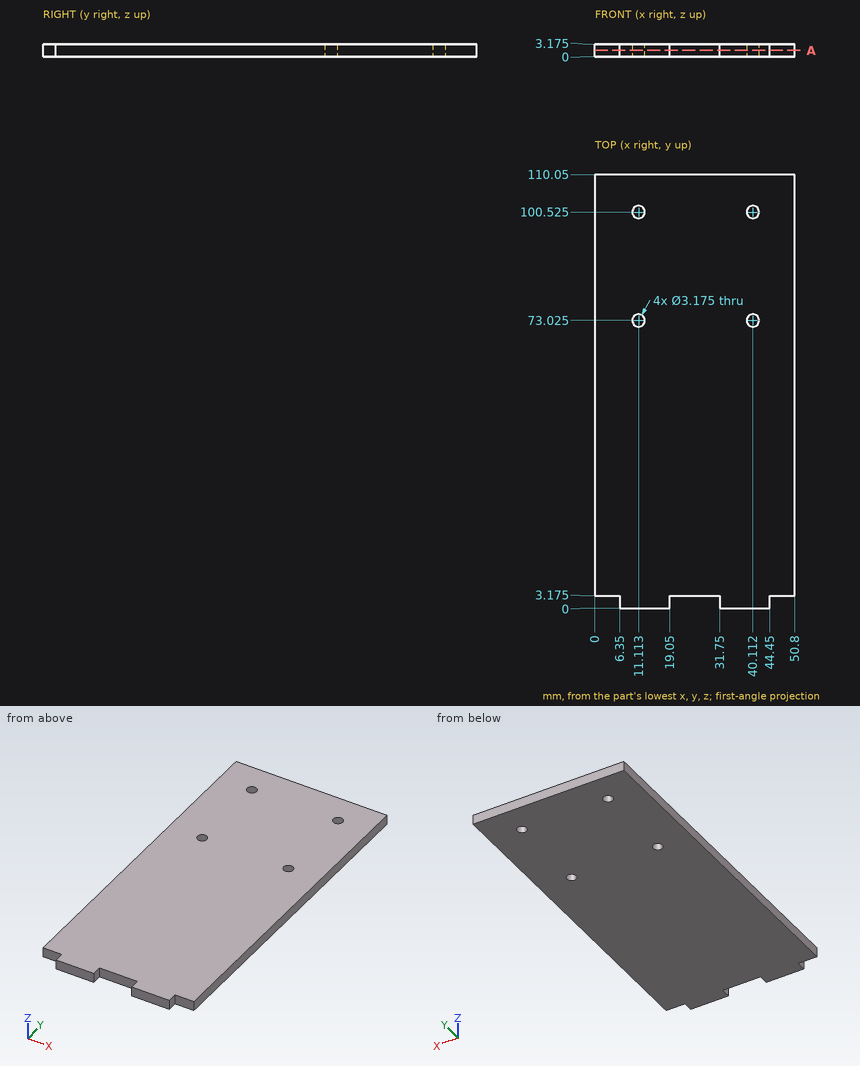
Part print with two shaded views. Sizes in mm from the minimum x, y, z corner. Round coordinates to 2 decimals unless told otherwise and drop trailing zeros.
(1) Pin check, flat tips, straight feed: pin 1 (1 mm diameter, centred on x = 28, z = 2, fed in from -Y) (1 decimal); pin 2 (1 mm diameter, centred on y = 1, z = 1.5, fed in from +X); pin 3 (1.6 mm diameter, centred on y = 2, z = 2, fed in from -X). Stop position of each tip, or through.
(2) Band-saw the part on A-A (z = 1.55). Give the number of separate pieces and of enclosed holes in the cut face, then the cut area to 3 significant figures.
(3) Drill centre line: line 1 (Y direction, x = 40, z = 1.1). Where is it in solid material? Low to high.
Verdict:
1. pin 1: stops at y = 3.2
1. pin 2: stops at x = 44.45
1. pin 3: stops at x = 6.35
2. separate pieces: 1
2. enclosed holes: 4
2. area: 5,480 mm2
3. line 1: y = 0 to 71.44, 74.61 to 98.94, 102.11 to 110.05
